Study the drawing (mm; zero at the part's minimum x, y, z) and answer. A direction names the side the tool comes from. Coordinates: 2 decimals unless noted, no trailing zeros. Order: outer loops, then holes, each group sorted by start corner. A loop starts at its lowest first (then second) coordinate and runs counter-clockwise, first axis right, second up.
1. Flat-ended cylindrical pins translate along their axes: pin 1 Ø4 at (x, y) = (21.5, 5) entering from -Z; pin 2 Ø4.5 at (x, z) = (19, 7) entering from +Y; pin 3 Ø2 at (y, z) = (12.5, 8) entering from +X. Find the tip coordinate at first contact, or state that the pin passes through.
2. A tool of negligible diameter and unlimited length cuts with its end or side. For the marked faces 1 and 2, from which of +Z, -Z, +X, -X, +Y, -Y can it reach the whole face along a straight path? Write none if from no direction.
3. The part is cut by section B-B, the plane y = 7.5. Give the vertices of the cut face in (x, z).
4. Find the intervals of material crossed by probe 1 along Y at (x, z) = (19.75, 12); probe 2 along X at (y, z) = (13.5, 10.25), in increasing order.
5. The part is cut by section A-A, the plane z = 8. Give the vertices of the cut face in (x, y), then the cut area to 3 significant figures.
6. The part is cut by section C-C, the plane x = 9.75. Give the vertices of the cut face in (y, z).
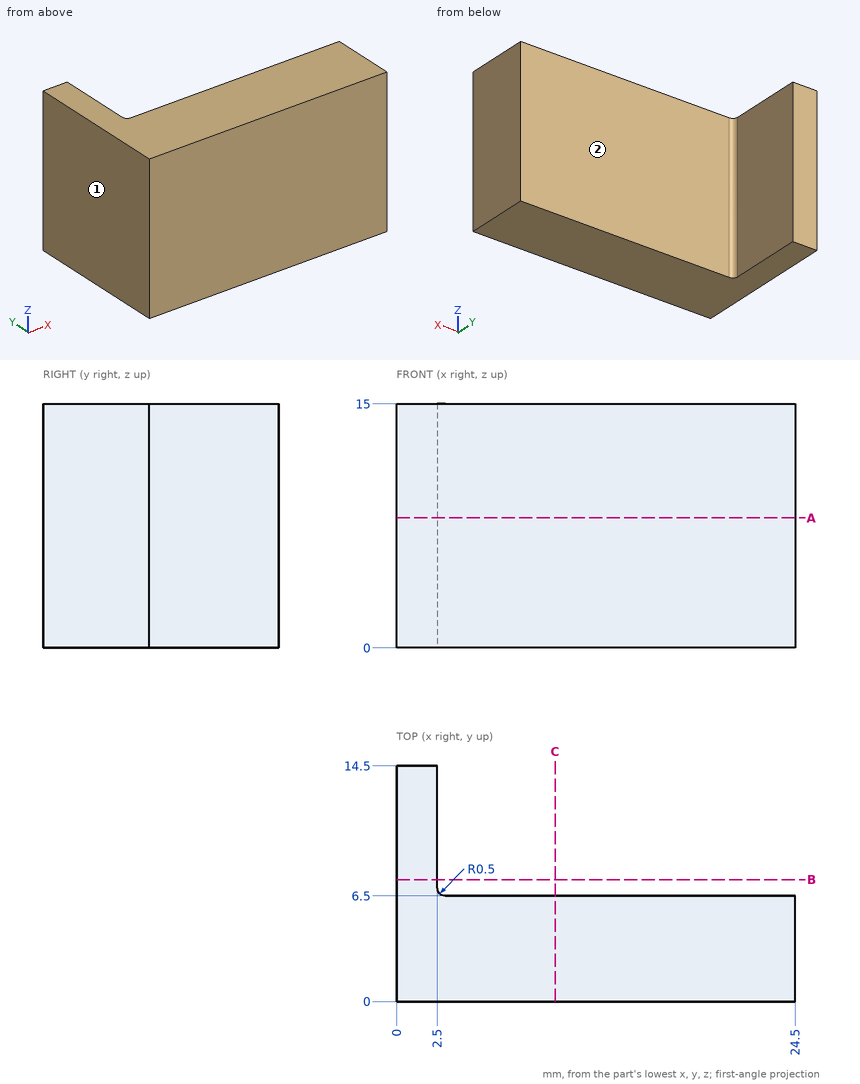
Geometry says:
1. pin 1: stops at z = 0
1. pin 2: stops at y = 6.5
1. pin 3: stops at x = 2.5
2. face 1: +Z, -Z, -X, +Y, -Y
2. face 2: +Z, -Z, +X, +Y
3. outline: (0, 0) - (2.5, 0) - (2.5, 15) - (0, 15) - close
4. probe 1: y = 0 to 6.5
4. probe 2: x = 0 to 2.5
5. outline: (0, 0) - (24.5, 0) - (24.5, 6.5) - (3, 6.5) arc R0.5 cw to (2.5, 7) - (2.5, 14.5) - (0, 14.5) - close
5. area: 179 mm2
6. outline: (0, 0) - (6.5, 0) - (6.5, 15) - (0, 15) - close
